```python
from build123d import *

# Parameters (mm, degrees)
BOSS_EXTRUDE1_DEPTH       = 12.7
SKETCH2_R                 = 2.4
CUT_EXTRUDE1_DEPTH        = 25.4
SKETCH2_3_R               = 3.1
CUT_EXTRUDE2_DEPTH        = 0.8
FILLET1_R                 = 3.6
SKETCH7_W                 = 25.4
SKETCH7_H                 = 38.1
BOSS_EXTRUDE2_DEPTH       = 6.35
F_8_CLEARANCE_HOLE1_D     = 4.4958
F_8_CLEARANCE_HOLE1_DEPTH = 6.35
BOSS_EXTRUDE3_DEPTH       = 1.5875
FILLET2_R                 = 6.35
FILLET3_R                 = 1.5875
FILLET4_R                 = 1.5875


# Some blends are built 0.0001 mm under size
with BuildPart() as part:
    # Sketch1 → Boss-Extrude1 (new, symmetric)
    with BuildSketch(Plane(origin=(0, 0, 0), x_dir=(1, 0, 0), z_dir=(0, 1, 0))):
        Polygon((0, 0), (0, -22.256250002), (-13.335, -22.256250002), (-13.335, -30.256250002), (6.35, -30.256250002), (6.35, 0), (15.875, 0), (15.875, 6.35), (-9.525, 6.35), (-9.525, 0), align=None)
    extrude(amount=BOSS_EXTRUDE1_DEPTH, both=True)

    # Sketch2 → Cut-Extrude1 (cut)
    with BuildSketch(Plane.XY.offset(30.256250002)):
        with BuildLine():
            ThreePointArc((-7.4722583, 0.73137085), (-7.367272665, 0), (-7.4722583, -0.73137085))
            Line((-7.4722583, -0.73137085), (-8.935, -0.73137085))
            Line((-8.935, -0.73137085), (-8.935, -2.19411255))
            ThreePointArc((-8.935, -2.19411255), (-9.735, -2.320249175), (-10.535, -2.19411255))
            Line((-10.535, -2.19411255), (-10.535, -0.73137085))
            Line((-10.535, -0.73137085), (-11.9977417, -0.73137085))
            ThreePointArc((-11.9977417, -0.73137085), (-12.102727335, 0), (-11.9977417, 0.73137085))
            Line((-11.9977417, 0.73137085), (-10.535, 0.73137085))
            Line((-10.535, 0.73137085), (-10.535, 2.19411255))
            ThreePointArc((-10.535, 2.19411255), (-9.735, 2.320249175), (-8.935, 2.19411255))
            Line((-8.935, 2.19411255), (-8.935, 0.73137085))
            Line((-8.935, 0.73137085), (-7.4722583, 0.73137085))
        make_face()
        with Locations((-9.735, -8)):
            Circle(SKETCH2_R)
        with Locations((-9.735, 8)):
            Circle(SKETCH2_R)
    extrude(amount=-CUT_EXTRUDE1_DEPTH, mode=Mode.SUBTRACT)

    # Sketch2<3> → Cut-Extrude2 (cut)
    with BuildSketch(Plane.XY.offset(30.256250002)):
        with Locations((-9.735, 8)):
            Circle(SKETCH2_3_R)
        with Locations((-9.735, -8)):
            Circle(SKETCH2_3_R)
    cut_extrude2 = extrude(amount=-CUT_EXTRUDE2_DEPTH, mode=Mode.SUBTRACT)

    # Mirror1: Cut-Extrude2 across plane
    add(cut_extrude2.mirror(Plane.XY.offset(26.256250002)), mode=Mode.SUBTRACT)

    # Fillet1
    fillet1_edges = [part.edges().sort_by_distance(p)[0] for p in [
        (-13.335, -12.7, 26.256250002),
        (-13.335, 12.7, 26.256250002),
    ]]
    fillet(fillet1_edges, radius=FILLET1_R)

    # Sketch7 → Boss-Extrude2 (add)
    with BuildSketch(Plane(origin=(0, 0, -6.35), x_dir=(-1, 0, 0), z_dir=(0, 0, -1))):
        with Locations((-3.175, -6.35)):
            Rectangle(SKETCH7_W, SKETCH7_H)
    extrude(amount=-BOSS_EXTRUDE2_DEPTH)

    # #8 Clearance Hole1
    with Locations(Plane(origin=(0, 0, -6.35), x_dir=(-1, 0, 0), z_dir=(0, 0, -1))):
        with Locations((-11.1125, 7.9375), (4.7625, 7.9375), (4.7625, -20.6375), (-11.1125, -20.6375)):
            Hole(F_8_CLEARANCE_HOLE1_D / 2, depth=F_8_CLEARANCE_HOLE1_DEPTH)

    # Sketch8 → Boss-Extrude3 (add, symmetric)
    with BuildSketch(Plane(origin=(3.175, 0, 0), x_dir=(0, 0, -1), z_dir=(1, 0, 0))):
        Polygon((0, -22.225), (-30.256250002, -12.7), (0, -12.7), align=None)
    extrude(amount=BOSS_EXTRUDE3_DEPTH, both=True)

    # Fillet2
    # the kernel refuses this fillet: 6.35 mm, written as the material it takes off along each edge
    with BuildSketch(Plane(origin=(6.35, -28.575, 30.256250002), x_dir=(-1, 0, 0), z_dir=(0, 1, 0))) as fillet2_piece_1:
        with BuildLine():
            CenterArc((FILLET2_R, -FILLET2_R), FILLET2_R, 90, 90)
            Line((0, -FILLET2_R), (0, 0))
            Line((0, 0), (FILLET2_R, 0))
        make_face()
    extrude(amount=57.15, mode=Mode.SUBTRACT)

    # Fillet3
    fillet3_edges = [part.edges().sort_by_distance(p)[0] for p in [
        (0, 0, 22.256250002),
    ]]
    fillet(fillet3_edges, radius=FILLET3_R)

    # Fillet4
    fillet4_edges = [part.edges().sort_by_distance(p)[0] for p in [
        (0, 0, 0),
        (6.35, 0, 0),
        (1.5875, -17.4625, 0),
        (4.7625, -17.4625, 0),
    ]]
    fillet(fillet4_edges, radius=FILLET4_R - 0.0001)  # a hair under: the kernel refuses the full size


solid = part.part
```
Geometry check sheet. Reference: the model listing, model coordinates, mm. A direction names the side the tool comes from. Round coordinates to 2 decimals unless told otherwise and drop trailing zeros. Loops run counter-clockwise (first coordinate to the right, second up) from the corner with the lowest first, then second, coordinate; pieces in that order, holes last. Notation, with made-up numbers: (6, 21) - (35, 21) arc R22 ccw to (35, 53) - close; hole circle Ø10 at (71.5, 8). An arc over 180 degrees is marked (long way). Write each question's results on one line, items separated by ' | '. Start each with the question number.
Q1. Access from +Z, -Z, +X, -X, +Y, -Y to the whole of each face (thin tool, end or side, straight path). Record for faces 1 (the flat face through (1.588, -16, 12)), 2 (the flat face through (-13.335, 0, 26)), 3 (the cylindrical face through (-9.75, 2.32, 26.31)), 4 (the flat face through (-8, 6, 23.056)), 5 (the cylindrical face through (-12.103, -0.01, 26.312)).
Q2. Cross-section at D-D on z = 27. Enter the section's corners in (x, y) (1 decimal).
Q3. Release check for a two-part mould opening along X. For faces 6 (the flat face through (4.762, -16, 12)), 7 (the flat face through (3, -25.4, -3)), 8 (the cylindrical face through (10.82, 10.166, -3.131)), 9 (the cylindrical face through (-0.45, -0.18, 0.48)) record: +X half, -X half, draft (parallel to the pull), parting line (faces both ways), or undercut.
Q4. Thickness scan on line 1 (Y direction, x = -9.25, z = 22.5); line 2 (Y direction, x = -4.25, z = -3.5); line 3 (X direction, y = -10, z = 16). Record the ranges inside material, lowest first. Write a range as [from, to].
Q5. Cross-section at B-B on x = -6. Enter the section's corners in (y, z), and give its area (3 significant figures).
Q6. Cross-section at C-C on x = -0.5. Enter the section's corners in (y, z), and give its area (3 significant figures).
Q7. Gauge pin test, flat ends, axial feed: P1, Ø21, axis at y = -5.5, z = 11.5, coming from the -X side; P2, Ø6, axis at x = 5, y = -5, coming from the +Z side; P3, Ø4, axis at y = -8, z = 19, coming from the -X side. Record the tip position at first contact, or that the pin passes through.
Answers below:
1) face 1: +Z, -X, -Y | face 2: +Z, -Z, -X, +Y, -Y | face 3: +Z | face 4: none | face 5: +Z, -Z
2) outline: (-13.3, -9.1) arc R3.6 ccw to (-9.7, -12.7) - (1.6, -12.7) - (1.6, -13.7) - (4.8, -13.7) - (4.8, -12.7) - (5.5, -12.7) - (5.5, 12.7) - (-9.7, 12.7) arc R3.6 ccw to (-13.3, 9.1) - close; hole circle Ø4.8 at (-9.7, -8); hole circle Ø4.8 at (-9.7, 8); hole (-12, -0.7) - (-10.5, -0.7) - (-10.5, -2.2) arc R2.6 ccw to (-8.9, -2.2) - (-8.9, -0.7) - (-7.5, -0.7) arc R2.6 ccw to (-7.5, 0.7) - (-8.9, 0.7) - (-8.9, 2.2) arc R2.6 ccw to (-10.5, 2.2) - (-10.5, 0.7) - (-12, 0.7) arc R2.6 ccw to start
3) face 6: +X half | face 7: draft | face 8: undercut | face 9: -X half
4) line 1: y = [-12.7, -11.06], [-4.94, -2.27], [2.27, 4.94], [11.06, 12.7] | line 2: y = [-25.4, -22.83], [-18.45, 5.75], [10.13, 12.7] | line 3: x = [0, 6.35]
5) outline: (-25.4, -6.35) - (-22.51, -6.35) - (-22.51, 0) - (-25.4, 0) - close; (-18.76, -6.35) - (6.06, -6.35) - (6.06, 0) - (-18.76, 0) - close; (-12.7, 22.26) - (12.7, 22.26) - (12.7, 30.26) - (-12.7, 30.26) - close; (9.81, -6.35) - (12.7, -6.35) - (12.7, 0) - (9.81, 0) - close | area: 397 mm²
6) outline: (-25.4, -6.35) - (12.7, -6.35) - (12.7, 0.43) - (-12.7, 0.43) - (-12.7, 0) - (-25.4, 0) - close; (-12.7, 21.83) - (12.7, 21.83) - (12.7, 30.26) - (-12.7, 30.26) - close | area: 467 mm²
7) P1: stops at x = -0.72 | P2: stops at z = 29.93 | P3: stops at x = -0.03
